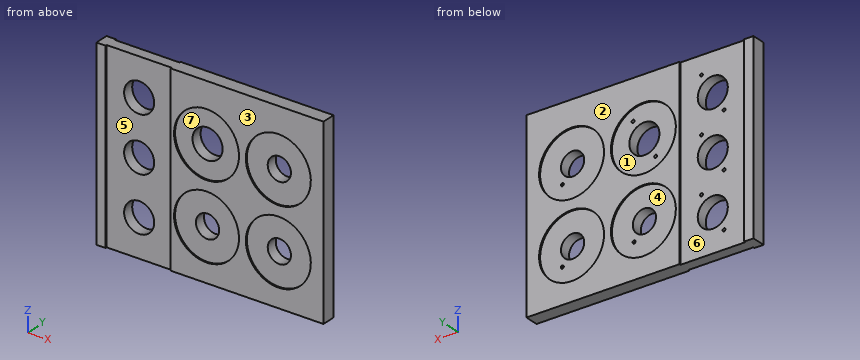
from build123d import *

# Parameters (mm, degrees)
SKETCH_1_W          = 332
SKETCH_1_H          = 270
EXTRUDE_1_DEPTH     = 20
SKETCH_2_W          = 95
SKETCH_2_H          = 289.731204414
CUT_EXTRUDE_1_DEPTH = 2
SKETCH_3_W          = 95
SKETCH_3_H          = 289.731204414
CUT_EXTRUDE_2_DEPTH = 2
CUT_EXTRUDE_3_REACH = 216.898
SKETCH_4_R          = 17
SKETCH_4_R_2        = 22
SKETCH_5_R          = 47.5
CUT_EXTRUDE_4_DEPTH = 2
CUT_EXTRUDE_START   = -2
SKETCH_6_R          = 47.5
CUT_EXTRUDE_5_DEPTH = 2
SKETCH_8_R          = 2.1
CUT_EXTRUDE_6_DEPTH = 12
SKETCH_9_R          = 2.25
CUT_EXTRUDE_7_DEPTH = 5


with BuildPart() as part:
    # 草图1 → 凸台-拉伸1 (new body)
    with BuildSketch(Plane(origin=(0, 0, 0), x_dir=(1, 0, 0), z_dir=(0, 1, 0))):
        Rectangle(SKETCH_1_W, SKETCH_1_H)
    extrude(amount=EXTRUDE_1_DEPTH)

    # 草图2 → 切除-拉伸1 (cut)
    with BuildSketch(Plane(origin=(0, 20, 0), x_dir=(1, 0, 0), z_dir=(0, 1, 0))):
        with Locations((-105, -0.900905486)):
            Rectangle(SKETCH_2_W, SKETCH_2_H)
    extrude(amount=-CUT_EXTRUDE_1_DEPTH, mode=Mode.SUBTRACT)

    # 草图3 → 切除-拉伸2 (cut)
    with BuildSketch(Plane.XZ):
        with Locations((-105, 0.900905486)):
            Rectangle(SKETCH_3_W, SKETCH_3_H)
    extrude(amount=-CUT_EXTRUDE_2_DEPTH, mode=Mode.SUBTRACT)

    # 草图4 → 切除-拉伸3 (cut, up to next)
    with BuildSketch(Plane(origin=(0, 20, 0), x_dir=(1, 0, 0), z_dir=(0, 1, 0)), mode=Mode.PRIVATE) as cut_extrude_3_sk1:
        with Locations(Location((-5, 60, 0), (0, 0, 270))):
            Circle(SKETCH_4_R)
    cut_extrude_3_tool1 = extrude(cut_extrude_3_sk1.sketch, amount=-CUT_EXTRUDE_3_REACH, mode=Mode.PRIVATE) & part.part
    # 草图4 → 切除-拉伸3 (cut, up to next)
    with BuildSketch(Plane(origin=(0, 20, 0), x_dir=(1, 0, 0), z_dir=(0, 1, 0)), mode=Mode.PRIVATE) as cut_extrude_3_sk2:
        with Locations(Location((-5, -50, 0), (0, 0, 270))):
            Circle(SKETCH_4_R_2)
    cut_extrude_3_tool2 = extrude(cut_extrude_3_sk2.sketch, amount=-CUT_EXTRUDE_3_REACH, mode=Mode.PRIVATE) & part.part
    # 草图4 → 切除-拉伸3 (cut, up to next)
    with BuildSketch(Plane(origin=(0, 20, 0), x_dir=(1, 0, 0), z_dir=(0, 1, 0)), mode=Mode.PRIVATE) as cut_extrude_3_sk3:
        with Locations(Location((100, -50, 0), (0, 0, 270))):
            Circle(SKETCH_4_R)
    cut_extrude_3_tool3 = extrude(cut_extrude_3_sk3.sketch, amount=-CUT_EXTRUDE_3_REACH, mode=Mode.PRIVATE) & part.part
    # 草图4 → 切除-拉伸3 (cut, up to next)
    with BuildSketch(Plane(origin=(0, 20, 0), x_dir=(1, 0, 0), z_dir=(0, 1, 0)), mode=Mode.PRIVATE) as cut_extrude_3_sk4:
        with Locations(Location((100, 60, 0), (0, 0, 270))):
            Circle(SKETCH_4_R)
    cut_extrude_3_tool4 = extrude(cut_extrude_3_sk4.sketch, amount=-CUT_EXTRUDE_3_REACH, mode=Mode.PRIVATE) & part.part
    # 草图4 → 切除-拉伸3 (cut, up to next)
    with BuildSketch(Plane(origin=(0, 20, 0), x_dir=(1, 0, 0), z_dir=(0, 1, 0)), mode=Mode.PRIVATE) as cut_extrude_3_sk5:
        with Locations(Location((-105, 80, 0), (0, 0, 270))):
            Circle(SKETCH_4_R_2)
    cut_extrude_3_tool5 = extrude(cut_extrude_3_sk5.sketch, amount=-CUT_EXTRUDE_3_REACH, mode=Mode.PRIVATE) & part.part
    # 草图4 → 切除-拉伸3 (cut, up to next)
    with BuildSketch(Plane(origin=(0, 20, 0), x_dir=(1, 0, 0), z_dir=(0, 1, 0)), mode=Mode.PRIVATE) as cut_extrude_3_sk6:
        with Locations(Location((-105, 0, 0), (0, 0, 270))):
            Circle(SKETCH_4_R_2)
    cut_extrude_3_tool6 = extrude(cut_extrude_3_sk6.sketch, amount=-CUT_EXTRUDE_3_REACH, mode=Mode.PRIVATE) & part.part
    # 草图4 → 切除-拉伸3 (cut, up to next)
    with BuildSketch(Plane(origin=(0, 20, 0), x_dir=(1, 0, 0), z_dir=(0, 1, 0)), mode=Mode.PRIVATE) as cut_extrude_3_sk7:
        with Locations(Location((-105, -80, 0), (0, 0, 270))):
            Circle(SKETCH_4_R_2)
    cut_extrude_3_tool7 = extrude(cut_extrude_3_sk7.sketch, amount=-CUT_EXTRUDE_3_REACH, mode=Mode.PRIVATE) & part.part
    add(cut_extrude_3_tool1.solids().sort_by_distance((-5, 20, -60))[0], mode=Mode.SUBTRACT)
    add(cut_extrude_3_tool2.solids().sort_by_distance((-5, 20, 50))[0], mode=Mode.SUBTRACT)
    add(cut_extrude_3_tool3.solids().sort_by_distance((100, 20, 50))[0], mode=Mode.SUBTRACT)
    add(cut_extrude_3_tool4.solids().sort_by_distance((100, 20, -60))[0], mode=Mode.SUBTRACT)
    add(cut_extrude_3_tool5.solids().sort_by_distance((-105, 20, -80))[0], mode=Mode.SUBTRACT)
    add(cut_extrude_3_tool6.solids().sort_by_distance((-105, 20, 0))[0], mode=Mode.SUBTRACT)
    add(cut_extrude_3_tool7.solids().sort_by_distance((-105, 20, 80))[0], mode=Mode.SUBTRACT)

    # 草图5 → 切除-拉伸4 (cut)
    with BuildSketch(Plane(origin=(0, 20, 0), x_dir=(1, 0, 0), z_dir=(0, 1, 0))):
        with Locations(Location((-5, 60, 0), (0, 0, 270))):
            Circle(SKETCH_5_R)
        with Locations(Location((100, 60, 0), (0, 0, 270))):
            Circle(SKETCH_5_R)
        with Locations(Location((100, -50, 0), (0, 0, 270))):
            Circle(SKETCH_5_R)
        with Locations(Location((-5, -50, 0), (0, 0, 270))):
            Circle(SKETCH_5_R)
    extrude(amount=-CUT_EXTRUDE_4_DEPTH, mode=Mode.SUBTRACT)

    # 草图6 → 切除-拉伸5 (cut)
    with BuildSketch(Plane.XZ.offset(CUT_EXTRUDE_START)):
        with Locations(Location((-5, -60, 0), (0, 0, 90))):
            Circle(SKETCH_6_R)
        with Locations(Location((100, -60, 0), (0, 0, 90))):
            Circle(SKETCH_6_R)
        with Locations(Location((100, 50, 0), (0, 0, 90))):
            Circle(SKETCH_6_R)
        with Locations(Location((-5, 50, 0), (0, 0, 90))):
            Circle(SKETCH_6_R)
    extrude(amount=CUT_EXTRUDE_5_DEPTH, mode=Mode.SUBTRACT)

    # 草图8 → 切除-拉伸6 (cut)
    with BuildSketch(Plane(origin=(0, 20, 0), x_dir=(1, 0, 0), z_dir=(0, 1, 0))):
        with Locations(Location((11.5, -78.578838325, 0), (0, 0, 270))):
            Circle(SKETCH_8_R)
        with Locations(Location((-21.5, -21.421161675, 0), (0, 0, 270))):
            Circle(SKETCH_8_R)
        with Locations(Location((-88.5, -108.578838325, 0), (0, 0, 270))):
            Circle(SKETCH_8_R)
        with Locations(Location((-88.5, -28.578838325, 0), (0, 0, 270))):
            Circle(SKETCH_8_R)
        with Locations(Location((-88.5, 51.421161675, 0), (0, 0, 270))):
            Circle(SKETCH_8_R)
        with Locations(Location((-121.5, 108.578838325, 0), (0, 0, 270))):
            Circle(SKETCH_8_R)
        with Locations(Location((-121.5, 28.578838325, 0), (0, 0, 270))):
            Circle(SKETCH_8_R)
        with Locations(Location((-121.5, -51.421161675, 0), (0, 0, 270))):
            Circle(SKETCH_8_R)
    extrude(amount=-CUT_EXTRUDE_6_DEPTH, mode=Mode.SUBTRACT)

    # 草图9 → 切除-拉伸7 (cut)
    with BuildSketch(Plane(origin=(0, 20, 0), x_dir=(1, 0, 0), z_dir=(0, 1, 0))):
        with Locations(Location((10, 83, 0), (0, 0, 270))):
            Circle(SKETCH_9_R)
        with Locations(Location((115, 83, 0), (0, 0, 270))):
            Circle(SKETCH_9_R)
        with Locations(Location((115, -27, 0), (0, 0, 270))):
            Circle(SKETCH_9_R)
    extrude(amount=-CUT_EXTRUDE_7_DEPTH, mode=Mode.SUBTRACT)


solid = part.part
Can you work these out from the model? Positions are in its coordinate system, mm. Face numbers are marked on the shaded views. A direction names the side the tool comes from. Give positions to 0.01 mm unless a question says otherwise; leave off trailing zeros. Write each loop counter-clockwise with the first axis right and the second up, starting at its lowest first coordinate (ties: lowest second). Pieces come first, ordered by that corner, then holes. Notation, with made-up numbers: (-11.75, 66) -> (8.25, 66) arc R18 cw to (8.25, 96) -> close; hole circle Ø9 at (-33, 2). An arc over 180 degrees is marked (long way). Answer as a JSON object with one key per item and string values. Group by question number.
Item 1: Suppose I cut it at A-A (x = -105). Please give me the cut outline in (y, z).
Item 2: Suppose I cut it at B-B (x = -5). Please give me the cut outline in (y, z), plus the area to 3 significant figures.
Item 3: Please list where these lines run through material, in increasing order: line 1 (X direction, y = 18.45, z = -60); line 2 (X direction, y = 9.25, z = 37); line 3 (X direction, y = 17.75, z = 45). Write a range as [from, to].
Item 4: Suppose I cut it at C-C (y = 12). State how many separate pieces and enclosed holes the cut face has, plus the area to 3 significant figures.
Item 5: We'd pull the mould along Z, two halves only. Please class the marked faces 1 and 2: +Z half, -Z half, draft (parallel to the pull), parting line (faces both ways), or undercut.
Item 6: I'm going to push flat-ended pins straight in: P1, Ø3.5, axis at x = -122.5, z = -28.5, coming from the +Y side; P2, Ø2.5, axis at x = -121.5, z = 51.42, coming from the +Y side; P3, Ø4, axis at x = -117, z = -104, coming from the -Y side. Where does each tip first touch, or does it pass through?
Item 7: Suppose I cut it at D-D (z = -114.5). Please give me the cut outline in (x, y).
Item 8: For the marked faces 3, 4, 5, 6 and 7, which set-ups out of +Z, -Z, +X, -X, +Y, -Y let a thin tool reach every point of the face, with its end or its side?
Findings:
{
 "1": {"outline": "(2, -135) -> (18, -135) -> (18, -102) -> (2, -102) -> close; (2, -58) -> (18, -58) -> (18, -22) -> (2, -22) -> close; (2, 22) -> (18, 22) -> (18, 58) -> (2, 58) -> close; (2, 102) -> (18, 102) -> (18, 135) -> (2, 135) -> close"},
 "2": {"outline": "(0, -135) -> (20, -135) -> (20, -107.5) -> (18, -107.5) -> (18, -77) -> (2, -77) -> (2, -107.5) -> (0, -107.5) -> close; (0, -12.5) -> (2, -12.5) -> (2, -43) -> (18, -43) -> (18, -12.5) -> (20, -12.5) -> (20, 2.5) -> (18, 2.5) -> (18, 28) -> (2, 28) -> (2, 2.5) -> (0, 2.5) -> close; (0, 97.5) -> (2, 97.5) -> (2, 72) -> (18, 72) -> (18, 97.5) -> (20, 97.5) -> (20, 135) -> (0, 135) -> close", "area": "3,390 mm²"},
 "3": {"line 1": "x = [-166, -152.5], [-57.5, -52.5], [42.5, 52.5], [147.5, 166]", "line 2": "x = [-166, -22.75], [12.75, 89.05], [110.95, 166]", "line 3": "x = [-166, -26.42], [16.42, 83.75], [116.25, 166]"},
 "4": {"separate pieces": "1", "enclosed holes": "15", "area": "80,700 mm²"},
 "5": {"face 1": "undercut", "face 2": "draft"},
 "6": {"P1": "stops at y = 18", "P2": "stops at y = 8", "P3": "stops at y = 2"},
 "7": {"outline": "(-166, 0) -> (-152.5, 0) -> (-152.5, 2) -> (-57.5, 2) -> (-57.5, 0) -> (166, 0) -> (166, 20) -> (-57.5, 20) -> (-57.5, 18) -> (-152.5, 18) -> (-152.5, 20) -> (-166, 20) -> close"},
 "8": {"face 3": "+Z, -Z, +X, -X, -Y", "face 4": "+Y", "face 5": "+Z, -Z, -Y", "face 6": "+Z, -Z, +Y", "face 7": "-Y"}
}
